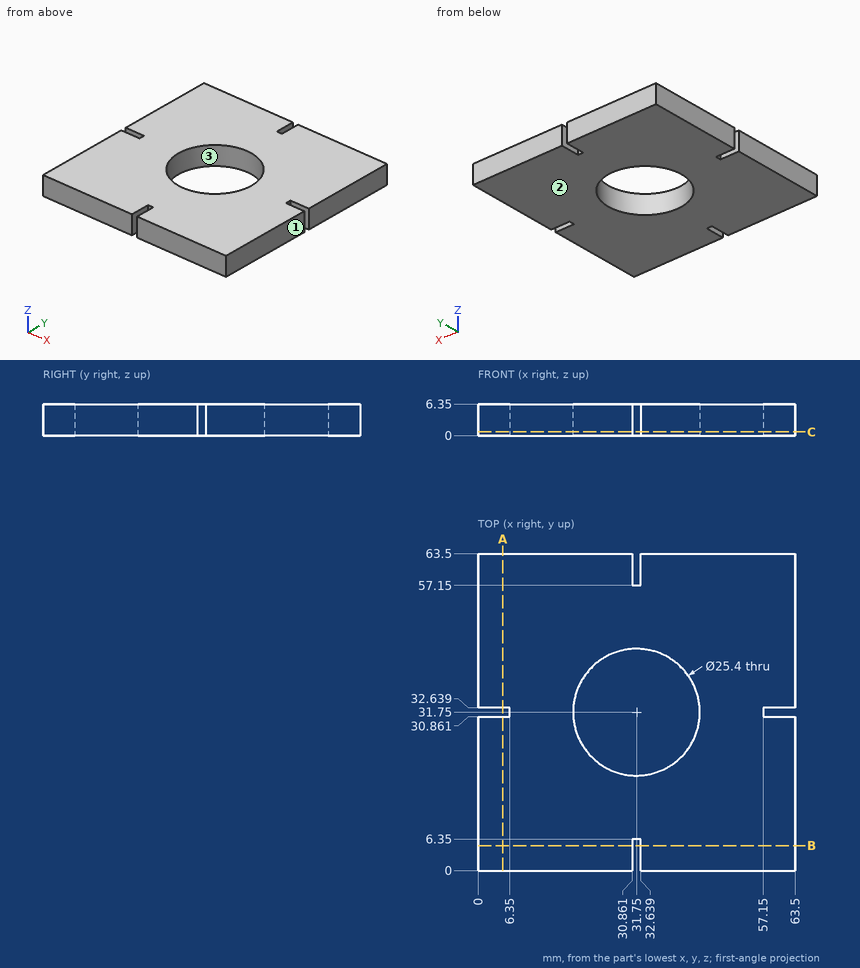
Geometry: see drawing. Coordinates: mm, zero at the bounding-box minimum. Round coordinates to 2 decimals unless told otherwise and drop trailing zeros. Write each loop counter-clockwise with the first axis right and the second up, starting at its lowest first coordinate (ties: lowest second). Pieces come first, ordered by that corner, then holes. Notation, with made-up numbers: M 88.5,0.25 L 144.5,0.25 A18 cw 144.5,28.25 Z; hole C 89,-21.75 d10. An arc over 180 degrees is marked long. Answer as a JSON object with one key per item and string values. Group by question number.
(1) Section query C-C on z = 0.75. Output: boundary loops of the cut face in (x, y), then the cut area to 3 significant figures.
(2) First-contact query: pin 1 (0.9 mm diameter, centred on y = 32, z = 3, fed in from +X). Flat tip, straight axial feed; report the tip coordinate or a pass-through.
(3) Section query A-A on x = 5. Output: boundary loops of the cut face in (y, z), then the cut area to 3 significant figures.
(4) Mould query, pull axis X, two halves, no side actions, for the marked faces 1, 2 and 3. Classes: +X half, -X half, draft (parallel to the pull), parting line (faces both ways), or undercut.
(5) Ray query, line 1 (X direction, y = 60, z = 2.25); line 2 (Y direction, x = 31.75, z = 3); line 3 (Y direction, x = 35, z = 4.5). Return the intervals inside material, ascending. Write a range as [from, to].
Computed values:
{
 "1": {"outline": "M 0,0 L 30.86,0 L 30.86,6.35 L 32.64,6.35 L 32.64,0 L 63.5,0 L 63.5,30.86 L 57.15,30.86 L 57.15,32.64 L 63.5,32.64 L 63.5,63.5 L 32.64,63.5 L 32.64,57.15 L 30.86,57.15 L 30.86,63.5 L 0,63.5 L 0,32.64 L 6.35,32.64 L 6.35,30.86 L 0,30.86 Z; hole C 31.75,31.75 d25.4", "area": "3,480 mm^2"},
 "2": {"pin 1": "x = 57.15"},
 "3": {"outline": "M 0,0 L 30.86,0 L 30.86,6.35 L 0,6.35 Z; M 32.64,0 L 63.5,0 L 63.5,6.35 L 32.64,6.35 Z", "area": "392 mm^2"},
 "4": {"face 1": "+X half", "face 2": "draft", "face 3": "undercut"},
 "5": {"line 1": "[0, 30.86], [32.64, 63.5]", "line 2": "[6.35, 19.05], [44.45, 57.15]", "line 3": "[0, 19.47], [44.03, 63.5]"}
}
